Model file for the job. Use its own axes, mm. A direction names the side the tool comes from. Coordinates: 2 decimals unless noted, no trailing zeros. Order: outer loops, then holes, each group sorted by start corner. A loop starts at its lowest first (then second) coordinate and runs counter-clockwise, first axis right, second up. Notation, with made-up numbers: (-19, 63.25) -> (5, 63.25) arc R28 ccw to (5, 99.25) -> close; hole circle Ø5 at (79, 76). An arc over 180 degrees is marked (long way). Use CSV: the item, a comma, the result in double quotes. Start each with the question number.
(1) Cut at B-B on y = 18. Write the cut outline in (x, z).
(2) Tool access for faces 4 (the cylindrical face through (-0.867, 8.246, 3.905)), 5 (the cylindrical face through (-0.5, 32.4, 2.4)), 6 (the flat face through (0, 28.6, 2)): list every direction of +Z, -Z, +X, -X, +Y, -Y with a clear straight run to the whole face (end or side of a thin tool).
(3) Cut at A-A on y = 24.5. Write the cut outline in (x, z).
(4) Pin check, flat tips, straight feed: pin 1 Ø1.5 at (x, z) = (1, 3) entering from +Y; pin 2 Ø4 at (x, z) = (3.5, -2.5) entering from +Y; pin 3 Ø1 at (x, z) = (3.5, 2.5) entering from +Y. Stop position of each tip, or through.
(5) Probe L1, parallel to Y at x = -2.75, z = 2.5; L2, parallel to X at y = 12, z = -2.5; L3, parallel to Y at x = 0.25, z = -2. List the from-to ranges inside material, lowest first.
(6) Pull direction Y, two halves, no side cores. Call faces 1 (the cylindrical face through (-0.29, 1.62, -2.23)), 2 (the flat face through (0, 0, 0)), 3 (the flat face through (0, 36, 0)): pulls with the +Y half, pulls with the -Y half, needs draft (parallel to the pull), parting line crosses it, or undercut.
```python
from build123d import *

# Parameters (mm, degrees)
SKETCH001_R  = 6
POCKET_DEPTH = 5
CHAMFER_SIZE = 0.5


with BuildPart() as part:
    # Sketch → Revolution (revolve)
    with BuildSketch(Plane.XY):
        Polygon((0, 0), (0, 36), (2.45, 36), (2.45, 29.35), (1.7, 29.35), (1.7, 28.6), (3.5, 28.6), (3.5, 23.5), (5.1, 23.5), (5.1, 19.75), (3.9, 19), (3.9, 11.4), (3, 11.4), (3, 8.5), (4, 8.5), (4, 8), (3.4, 8), (2.665, 7.15), (2.665, 6.5), (2.25, 6.5), (2.25, 5.75), (2.665, 5.75), (2.665, 2), (2.25, 2), (2.25, 1.25), (2.665, 1.25), (2.665, 0), align=None)
    revolve(axis=Axis((0, 0, 0), (0, 1, 0)))

    # Sketch001 (on DatumPlane) → Pocket (cut)
    with BuildSketch(Plane(origin=(0, 23.5, 0), x_dir=(-1, 0, 0), z_dir=(0, 1, 0))):
        Circle(SKETCH001_R)
        Polygon((4.41673, 2.55), (0, 5.1), (-4.41673, 2.55), (-4.41673, -2.55), (0, -5.1), (4.41673, -2.55), align=None, mode=Mode.SUBTRACT)
    extrude(amount=-POCKET_DEPTH, mode=Mode.SUBTRACT)

    # Chamfer
    chamfer_edges = [part.edges().sort_by_distance(p)[0] for p in [
        (4.158365, 19.161478, 0),
        (2.25, 1.625, 0),
        (-3.5, 28.6, 0),
        (-2.45, 36, 0),
    ]]
    chamfer(chamfer_edges, length=CHAMFER_SIZE)


solid = part.part
```
Outcome:
1,outline,"circle Ø7.8 at (0, 0)"
2,face 4,"-Y"
2,face 5,"+Y"
2,face 6,"none"
3,outline,"circle Ø7 at (0, 0)"
4,pin 1,"y = 35.54"
4,pin 2,"y = 35.65"
4,pin 3,"y = 23.5"
5,L1,"8 to 8.5, 11.4 to 23.5"
5,L2,"-2.99 to 2.99"
5,L3,"0 to 28.6, 29.35 to 35.93"
6,face 1,"undercut"
6,face 2,"pulls with the -Y half"
6,face 3,"pulls with the +Y half"
